Work out the finished part from the listing and answer in its coordinate system (mm). Give positions to 0.01 mm unless a question says otherwise; leave off trailing zeros. Order: outer loops, then holes, each group sorted by start corner. A loop starts at its lowest first (then second) coordinate and runs counter-clockwise, first axis right, second up. Notation, with made-up numbers: (77, 32.25) - (118, 32.25) arc R18 ccw to (118, 58.25) - close; hole circle Ø3 at (18, 54.25). An arc over 180 degrees is marked (long way). Put each result on its own line as item: value.
```python
from build123d import *

# Parameters (mm, degrees)
SKETCH4_R          = 2.38125
CUT_EXTRUDE2_DEPTH = 6.35
FILLET1_R          = 0.396875
CHAMFER1_SIZE      = 0.762


with BuildPart() as part:
    # Sketch1 → Revolve1 (revolve)
    with BuildSketch(Plane(origin=(0, 0, 0), x_dir=(1, 0, 0), z_dir=(0, 1, 0))):
        with BuildLine():
            Line((1.5875, 0), (9.525, 0))
            ThreePointArc((9.525, 0), (7.274838916, 6.148361062), (1.5875, 9.391776656))
            Line((1.5875, 9.391776656), (1.5875, 0))
        make_face()
    revolve(axis=Axis((0, 0, 0), (0, 0, -1)))

    # Sketch4 → Cut-Extrude2 (cut)
    with BuildSketch(Plane(origin=(0, 0, -9.525), x_dir=(-1, 0, 0), z_dir=(0, 0, -1))):
        Circle(SKETCH4_R)
    extrude(amount=-CUT_EXTRUDE2_DEPTH, mode=Mode.SUBTRACT)

    # Fillet1
    fillet1_edges = [part.edges().sort_by_distance(p)[0] for p in [
        (2.38125, 0, -3.175),
    ]]
    fillet(fillet1_edges, radius=FILLET1_R)

    # Chamfer1
    # the kernel refuses this chamfer: 0.762 mm, written as the material it takes off along each edge
    with BuildSketch(Plane(origin=(0, 0, 0), x_dir=(1, 0, 0), z_dir=(0, 1, 0))) as chamfer1_piece_1:
        with BuildLine():
            Line((9.525 - CHAMFER1_SIZE, 0), (9.496699923, 0.733699923))
            ThreePointArc((9.496699923, 0.733699923), (9.517517871, 0.37746333), (9.525, 0))
            Line((9.525, 0), (9.525 - CHAMFER1_SIZE, 0))
        make_face()
    revolve(axis=Axis((0, 0, 0), (0, 0, -1)), mode=Mode.SUBTRACT)

    # Chamfer2: read off the stored shape, not the designer's step
    # Chamfer2 outline → Chamfer2 (revolve, cut)
    with BuildSketch(Plane.XZ):
        Polygon((2.033114035, -3.178004117), (1.5875, -2.673849388), (1.5875, -3.178004117), align=None)
        Polygon((1.5875, 0), (1.5875, -0.508), (2.0955, 0), align=None)
        Polygon((2.857431183, -9.086292535), (2.38125, -8.805548582), (2.38125, -9.086292535), align=None)
    revolve(axis=Axis((0, 0, 0), (0, 0, 1)), mode=Mode.SUBTRACT)

    # Chamfer2 2 outline → Chamfer2 2 (revolve, cut)
    with BuildSketch(Plane.XZ):
        with BuildLine():
            Line((2.857431193, -9.086292532), (2.38125, -9.086292535))
            Line((2.38125, -9.086292535), (2.381249991, -9.222541596))
            ThreePointArc((2.381249991, -9.222541596), (2.620226343, -9.157512703), (2.857431193, -9.086292532))
        make_face()
    revolve(axis=Axis((0, 0, 0), (0, 0, 1)), mode=Mode.SUBTRACT)


solid = part.part
```
(1) Section D-D, the plane z = -1 is taken. Write down the section's boundary in (x, y) (1 decimal), then the cut area to 3 significant figures.
Geometry check:
outline: circle Ø18.9 at (0, 0); hole circle Ø3.2 at (0, 0)
area: 274 mm²
(2) Straight lines are drawn through the part: line 1 (Y direction, x = 0, z = -2.05); line 2 (Y direction, x = 0, z = -5.05); line 3 (X direction, y = 0, z = -7.3). For each, find the intervals that lie inside material, in ascending order.
Geometry check:
line 1: y = -9.3 to -1.59, 1.59 to 9.3
line 2: y = -8.08 to -2.38, 2.38 to 8.08
line 3: x = -6.12 to -2.38, 2.38 to 6.12
(3) Given pin 1 (3 mm diameter, centred on x = -6, z = -8, fed in from +Y); pin 2 (5 mm diameter, centred on y = -7, z = -5.5, fed in from +X); pin 3 (5 mm diameter, centred on y = 5.5, z = -5.5, fed in from +X), each flat-ended and moving along its own axis, determine where each tip first touches the part or whether it passes through.
Geometry check:
pin 1: stops at y = 4.3
pin 2: stops at x = 7.05
pin 3: stops at x = 7.93
(4) Determine the mould class of faces 1 (the face through (-2, 2, 0)), 2 (the face through (1.89, -1.45, -6.23)) for opening direction Y: pulls with the +Y half, pulls with the -Y half, needs draft (parallel to the pull), parting line crosses it, or undercut.
Geometry check:
face 1: needs draft
face 2: undercut
(5) Section C-C, the plane z = -8.25 is taken. Write down the section's boundary in (x, y).
Geometry check:
outline: circle Ø9.52 at (0, 0); hole circle Ø4.76 at (0, 0)
